Autodesk Inventor part; units mm, degrees
ref_plane "Work Plane1" through (0, 0, 0) normal (1, 0, 0) x (0, 0, 1)
ref_plane "XZ Plane" through (0, 0, 0) normal (0, 1, 0) x (-1, 0, 0)
ref_plane "XY Plane" through (0, 0, 0) normal (0, 0, 1) x (1, 0, 0)
sketch "Sketch1" plane through (0, 0, 0) normal (0, 0, 1) x (1, 0, 0)
  circle A0 centre (0, 0) radius 13.0969
  circle A1 centre (0, 0) radius 16.6688
  dimension "d0" = 26.1938
  dimension "d1" = 33.3375
extrude "Extrusion1" add sketch "Sketch1" along normal blind 355.6
ref_plane "Work Plane1" through (0, 0, 0) normal (1, 0, 0) x (0, 0, 1)
sketch "Sketch2" plane through (0, 0, 0) normal (1, 0, 0) x (0, 0, 1)
  circle A0 centre (146.05, 0) radius 2.4257
  line L0 (-71.12, 0) -> (426.72, 0)
  line L1 (355.6, 13.0969) -> (355.6, -13.0969)
  dimension "d5" = 4.8514
  dimension "d6" = 209.55
extrude "Extrusion2" cut sketch "Sketch2" against normal mid plane 381
pattern_linear "Rectangular Pattern1" count 2 spacing 50.8 along (0, 0, -1) of "Extrusion2"
properties part number "FE-00026"
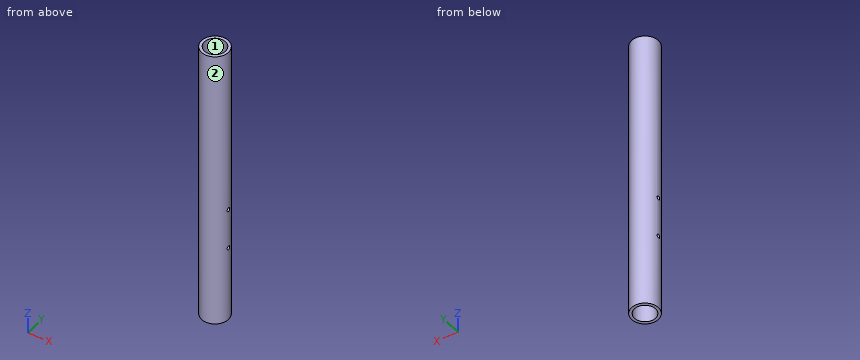
Read the model definition and answer for the solid it produces. Units are mm, in the model's axes. Face numbers are marked on the shaded views. Give positions to 0.01 mm unless a question says otherwise; leave off trailing zeros. Write each loop counter-clockwise with the first axis right and the second up, starting at its lowest first coordinate (ties: lowest second). Pieces come first, ordered by that corner, then holes. Notation, with made-up numbers: (74.5, 55) -> (87.5, 55) arc R18 cw to (87.5, 83) -> close; hole circle Ø7 at (25.25, 53). An arc over 180 degrees is marked (long way). Answer as a JSON object with one key per item and string values.
1) Straight lines are drawn through the part: probe 1 along Z at (x, y) = (14.7, 0); probe 2 along X at (y, z) = (0, 247). For each, find the intervals that lie inside material, in ascending order. Write a range as from..to.
Findings below:
{"probe 1": "z = 0..92.82, 97.68..143.62, 148.48..355.6", "probe 2": "x = -16.67..-13.1, 13.1..16.67"}
2) Flat-ended cylindrical pins translate along their axes: pin 1 Ø5 at (x, y) = (12.5, 4.5) entering from -Z; pin 2 Ø4 at (x, z) = (4.5, 317) entering from +Y; pin 3 Ø4 at (y, z) = (0, 95.25) entering from +X; pin 4 Ø3 at (x, z) = (12.5, 211.5) entering from -Y. Find the tip coordinate at first contact, or state that the pin passes through.
Findings below:
{"pin 1": "stops at z = 0", "pin 2": "stops at y = 16.48", "pin 3": "passes through", "pin 4": "stops at y = -12.52"}
3) Section B-B on z = 180.5 is taken. Write down the section's boundary in (x, y), then the cut area to 3 significant figures.
Findings below:
{"outline": "circle Ø33.34 at (0, 0); hole circle Ø26.19 at (0, 0)", "area": "334 mm^2"}
4) Section A-A on x = -3 is taken. Write down the section's boundary in (y, z).
Findings below:
{"outline": "(-16.4, 0) -> (-12.75, 0) -> (-12.75, 355.6) -> (-16.4, 355.6) -> close; (12.75, 0) -> (16.4, 0) -> (16.4, 355.6) -> (12.75, 355.6) -> close"}
5) For a pull along X with two mould halves and no side action, classify the marked faces 1 and 2 as pulls with the +X half, pulls with the -X half, needs draft (parallel to the pull), parting line crosses it, or undercut.
Findings below:
{"face 1": "undercut", "face 2": "parting line crosses it"}
